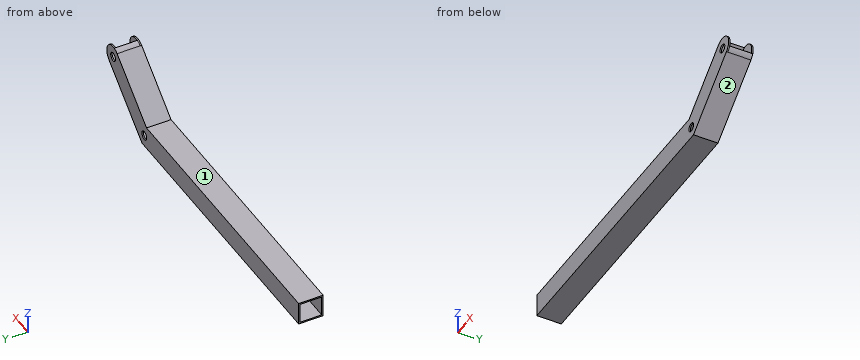
from build123d import *

# Parameters (mm, degrees)
BOSS_EXTRUDE1_DEPTH = 1.5875
BOSS_EXTRUDE2_DEPTH = 25.4
BOSS_EXTRUDE3_START = -1.5875
BOSS_EXTRUDE3_DEPTH = 1.5875
SKETCH7_R           = 4.826
CUT_EXTRUDE1_DEPTH  = 45.2755


with BuildPart() as part:
    # Sketch1 → Boss-Extrude1 (new body)
    with BuildSketch(Plane(origin=(0, 0, 0), x_dir=(1, 0, 0), z_dir=(0, 1, 0))):
        with BuildLine():
            Line((167.59049564, -102.48416143), (107.894507528, -52.393279822))
            Line((107.894507528, -52.393279822), (-200.411070496, -52.393279822))
            Line((-200.411070496, -52.393279822), (-200.411070496, -26.993279822))
            Line((-200.411070496, -26.993279822), (117.139351479, -26.993279822))
            Line((117.139351479, -26.993279822), (183.917300926, -83.026632574))
            ThreePointArc((183.917300926, -83.026632574), (185.482662711, -100.918799645), (167.59049564, -102.48416143))
        make_face()
    extrude(amount=BOSS_EXTRUDE1_DEPTH)

    # Sketch2 → Boss-Extrude2 (add)
    with BuildSketch(Plane(origin=(0, 1.5875, 0), x_dir=(1, 0, 0), z_dir=(0, 1, 0))):
        with BuildLine():
            Line((187.606793422, -88.194818438), (117.139351479, -29.065613894))
            Line((117.139351479, -29.065613894), (117.139351479, -28.580779822))
            Line((117.139351479, -28.580779822), (116.561548732, -28.580779822))
            Line((116.561548732, -28.580779822), (116.118926148, -28.209375376))
            Line((116.118926148, -28.209375376), (115.807280814, -28.580779822))
            Line((115.807280814, -28.580779822), (-200.411070496, -28.580779822))
            Line((-200.411070496, -28.580779822), (-200.411070496, -26.993279822))
            Line((-200.411070496, -26.993279822), (117.139351479, -26.993279822))
            Line((117.139351479, -26.993279822), (183.917300926, -83.026632574))
            ThreePointArc((183.917300926, -83.026632574), (186.090270011, -85.376412011), (187.606793422, -88.194818438))
        make_face()
        with BuildLine():
            Line((-200.411070496, -52.393279822), (-200.411070496, -50.805779822))
            Line((-200.411070496, -50.805779822), (108.472310275, -50.805779822))
            Line((108.472310275, -50.805779822), (173.320838796, -105.220156187))
            ThreePointArc((173.320838796, -105.220156187), (170.281908769, -104.216083315), (167.59049564, -102.48416143))
            Line((167.59049564, -102.48416143), (107.894507528, -52.393279822))
            Line((107.894507528, -52.393279822), (-200.411070496, -52.393279822))
        make_face()
    extrude(amount=BOSS_EXTRUDE2_DEPTH)

    # Sketch6 → Boss-Extrude3 (add)
    with BuildSketch(Plane(origin=(0, 26.9875, 0), x_dir=(1, 0, 0), z_dir=(0, 1, 0)).offset(BOSS_EXTRUDE3_START)):
        with BuildLine():
            Line((-200.411070496, -26.993279822), (117.139351479, -26.993279822))
            Line((117.139351479, -26.993279822), (183.917300926, -83.026632574))
            ThreePointArc((183.917300926, -83.026632574), (185.482662711, -100.918799645), (167.59049564, -102.48416143))
            Line((167.59049564, -102.48416143), (107.894507528, -52.393279822))
            Line((107.894507528, -52.393279822), (-200.411070496, -52.393279822))
            Line((-200.411070496, -52.393279822), (-200.411070496, -26.993279822))
        make_face()
    extrude(amount=BOSS_EXTRUDE3_DEPTH)

    # Sketch7 → Cut-Extrude1 (cut)
    with BuildSketch(Plane(origin=(0, 26.9875, 0), x_dir=(1, 0, 0), z_dir=(0, 1, 0))):
        with Locations(Location((175.753898283, -92.755397002, 0), (0, 0, 270))):
            Circle(SKETCH7_R)
        with Locations(Location((112.516929504, -39.693279822, 0), (0, 0, 270))):
            Circle(SKETCH7_R)
    extrude(amount=-CUT_EXTRUDE1_DEPTH, mode=Mode.SUBTRACT)


solid = part.part
The model under review builds one solid part; all positions refer to its coordinate system, in mm. Face numbers are marked on the shaded views. A direction names the side the tool comes from. Round coordinates to 2 decimals unless told otherwise and drop trailing zeros. Loops run counter-clockwise (first coordinate to the right, second up) from the corner with the lowest first, then second, coordinate; pieces in that order, holes last. Notation, with made-up numbers: (8, 19) -> (15, 19) arc R12 cw to (15, 42) -> close; hole circle Ø9 at (26.25, 43.25). An arc over 180 degrees is marked (long way). One line per question, with ' | ' between items. Start each with the question number.
Item 1: Machinability: for the marked faces 1 and 2, which of the approach directions +Z, -Z, +X, -X, +Y, -Y give a long, thin tool a straight path to every point of the face, cutting with its end or side? Answer none if there is none.
Item 2: Wall thickness on line 1 along Y through (x, z) = (4, 46.5); line 2 along Z through (x, y) = (83, 24); line 3 along X through (y, z) = (3, 73): over which ranges is each line inside the solid? List them lowest first. Write a range as [from, to].
Item 3: Add section D-D, the plane z = 57. Write out the cut boundary in (x, y), then the cut area to 3 significant figures.
Item 4: Add section A-A, the plane y = 16.5. Write out the cut boundary in (x, z), then the cut area to 3 significant figures.
Item 5: For pin 1 (2 mm diameter, centred on x = 139, y = 22.5, fed in from +Z); pin 2 (13.5 mm diameter, centred on x = 26.5, y = 19.5, fed in from +Z); pin 3 (7.5 mm diameter, centred on x = 175.75, z = 92.76, fed in from +Y); pin 4 (0.5 mm diameter, centred on x = 116.5, y = 9.5, fed in from +Z), all flat-tipped, find the tip position at first contact; note any pin that passes through.
Item 6: Add section B-B, the plane x = -42.5. Write out the cut boundary in (y, z).
Item 7: Add section C-C, the plane z = 39. Write out the cut boundary in (x, y), then the cut area to 3 significant figures.
Return value:
1) face 1: +Z, -X, +Y, -Y | face 2: -Z, +X, +Y, -Y
2) line 1: y = [0, 1.59], [25.4, 26.99] | line 2: z = [26.99, 28.58], [50.81, 52.39] | line 3: x = [132.45, 134.92], [169.5, 171.97]
3) outline: (113.38, 0) -> (152.9, 0) -> (152.9, 26.99) -> (113.38, 26.99) -> close; hole (115.85, 1.59) -> (150.43, 1.59) -> (150.43, 25.4) -> (115.85, 25.4) -> close | area: 243 mm2
4) outline: (-200.41, 26.99) -> (117.14, 26.99) -> (183.92, 83.03) arc R12.7 ccw to (187.61, 88.19) -> (117.14, 29.07) -> (117.14, 28.58) -> (116.56, 28.58) -> (116.12, 28.21) -> (115.81, 28.58) -> (-200.41, 28.58) -> close; (-200.41, 50.81) -> (108.47, 50.81) -> (173.32, 105.22) arc R12.7 ccw to (167.59, 102.48) -> (107.89, 52.39) -> (-200.41, 52.39) -> close | area: 1,270 mm2
5) pin 1: stops at z = 79.33 | pin 2: stops at z = 52.39 | pin 3: passes through | pin 4: stops at z = 59.82
6) outline: (0, 26.99) -> (26.99, 26.99) -> (26.99, 52.39) -> (0, 52.39) -> close; hole (1.59, 28.58) -> (25.4, 28.58) -> (25.4, 50.81) -> (1.59, 50.81) -> close
7) outline: (-200.41, 0) -> (107.74, 0) -> (107.74, 1.59) -> (-200.41, 1.59) -> close; (-200.41, 25.4) -> (107.74, 25.4) -> (107.74, 26.99) -> (-200.41, 26.99) -> close; (117.29, 0) -> (131.45, 0) -> (131.45, 26.99) -> (117.29, 26.99) -> (117.29, 25.4) -> (128.98, 25.4) -> (128.98, 1.59) -> (117.29, 1.59) -> close | area: 1,080 mm2
